CAD build for the part. Positions are in the model's coordinates, mm. Face numbers are marked on the shaded views. A direction names the side the tool comes from. Give positions to 0.01 mm unless a question says otherwise; leave off trailing zeros. Write each loop counter-clockwise with the first axis right and the second up, starting at its lowest first coordinate (ties: lowest second). Pieces come first, ordered by that corner, then holes. Notation, with made-up numbers: (85, -7.5) - (105, -7.5) arc R34 cw to (105, 23.5) - close; hole circle Ø3 at (-11, 85). An arc over 180 degrees is marked (long way). Put each result on its own line as item: value. Start each with the question number.
1. Tool access for the marked faces 4, 5 and 6: list every direction of +Z, -Z, +X, -X, +Y, -Y with a clear straight run to the whole face (end or side of a thin tool).
2. Mould opens along Y. For the marked faces 1, 2 and 3 say: +Y half, -Y half, draft (parallel to the pull), parting line (faces both ways), or undercut.
3. Drop flat-ended pins along their axis: pin 1 (2 mm diameter, centred on x = 5, z = 1.5, fed in from +Y); pin 2 (2 mm diameter, centred on x = -2.5, y = 4.5, fed in from +Z); pin 3 (8 mm diameter, centred on x = 4.5, y = 28.5, fed in from +Z); pin 4 (7 mm diameter, centred on y = 53.5, z = 0, fed in from +X). Give the stop position or say it passes through.
4. Cut at B-B on z = -4.25. List the corners of the cut face in (x, y), and give its area (3 significant figures).
5. Cut at D-D on y = 13.5. List the corners of the cut face in (x, z), and give its area (3 significant figures).
6. Cut at C-C on x = 3.25. List the corners of the cut face in (y, z), and give its area (3 significant figures).
7. Wall check: line 1 (Y direction, x = 5.2, z = 0); line 2 (Z direction, x = 3.65, y = 53.5); line 3 (Y direction, x = 6.25, z = 4.25). Give the ranges that are in metal, low to high.
8. Cut at A-A on x = -4.5. List the corners of the cut face in (y, z).
from build123d import *

# Parameters (mm, degrees)
SKETCH1_R           = 7.5
BOSS_EXTRUDE1_DEPTH = 46
SKETCH2_W           = 15
SKETCH2_H           = 15
BOSS_EXTRUDE2_DEPTH = 10
SKETCH3_R           = 2.5
CUT_EXTRUDE1_DEPTH  = 7.5
BOSS_EXTRUDE3_DEPTH = 15
CUT_EXTRUDE4_DEPTH  = 64.263338514
SKETCH6_R           = 6
CUT_EXTRUDE5_DEPTH  = 64.263338514
CUT_EXTRUDE7_START  = -5
SKETCH7_R           = 7.5
CUT_EXTRUDE7_DEPTH  = 5
CUT_EXTRUDE8_START  = -5
CUT_EXTRUDE8_DEPTH  = 5


with BuildPart() as part:
    # Sketch1 → Boss-Extrude1 (new body)
    with BuildSketch(Plane(origin=(0, 0, 0), x_dir=(1, 0, 0), z_dir=(0, 1, 0))):
        with Locations(Location((0, 0, 0), (0, 0, 270))):
            Circle(SKETCH1_R)
    extrude(amount=BOSS_EXTRUDE1_DEPTH)

    # Sketch2 → Boss-Extrude2 (add)
    with BuildSketch(Plane.XZ):
        Rectangle(SKETCH2_W, SKETCH2_H)
    extrude(amount=BOSS_EXTRUDE2_DEPTH)

    # Sketch3 → Cut-Extrude1 (cut)
    with BuildSketch(Plane.ZY.offset(7.5)):
        with Locations((0, -5)):
            Circle(SKETCH3_R)
    extrude(amount=-CUT_EXTRUDE1_DEPTH, mode=Mode.SUBTRACT)

    # Sketch4 → Boss-Extrude3 (add)
    with BuildSketch(Plane(origin=(0, 46, 0), x_dir=(1, 0, 0), z_dir=(0, 1, 0))):
        Polygon((0, 7.5), (7.5, 7.5), (7.5, -7.5), (-7.5, -7.5), (-7.5, 7.5), align=None)
    extrude(amount=BOSS_EXTRUDE3_DEPTH)

    # Sketch5 → Cut-Extrude4 (cut, through all)
    with BuildSketch(Plane.ZY.offset(7.5)):
        with BuildLine():
            ThreePointArc((-7.5, 53.5), (-5.303300859, 58.803300859), (0, 61))
            Line((0, 61), (-7.5, 61))
            Line((-7.5, 61), (-7.5, 53.5))
        make_face()
        with BuildLine():
            Line((7.5, 61), (0, 61))
            ThreePointArc((0, 61), (5.303300859, 58.803300859), (7.5, 53.5))
            Line((7.5, 53.5), (7.5, 61))
        make_face()
    extrude(amount=-CUT_EXTRUDE4_DEPTH, mode=Mode.SUBTRACT)

    # Sketch6 → Cut-Extrude5 (cut, through all)
    with BuildSketch(Plane.ZY.offset(7.5)):
        with Locations((0, 53.5)):
            Circle(SKETCH6_R)
    extrude(amount=-CUT_EXTRUDE5_DEPTH, mode=Mode.SUBTRACT)

    # Sketch7 → Cut-Extrude7 (cut)
    with BuildSketch(Plane.ZY.offset(7.5).offset(CUT_EXTRUDE7_START)):
        with Locations((0, 53.5)):
            Circle(SKETCH7_R)
    extrude(amount=-CUT_EXTRUDE7_DEPTH, mode=Mode.SUBTRACT)

    # Sketch8 → Cut-Extrude8 (cut)
    with BuildSketch(Plane.ZY.offset(7.5).offset(CUT_EXTRUDE8_START)):
        with BuildLine():
            Line((-6, 53.5), (-7.5, 53.5))
            Line((-7.5, 53.5), (-7.5, 46))
            Line((-7.5, 46), (0, 46))
            Line((0, 46), (7.5, 46))
            Line((7.5, 46), (7.5, 53.5))
            Line((7.5, 53.5), (6, 53.5))
            ThreePointArc((6, 53.5), (0, 47.5), (-6, 53.5))
        make_face()
    extrude(amount=-CUT_EXTRUDE8_DEPTH, mode=Mode.SUBTRACT)


solid = part.part
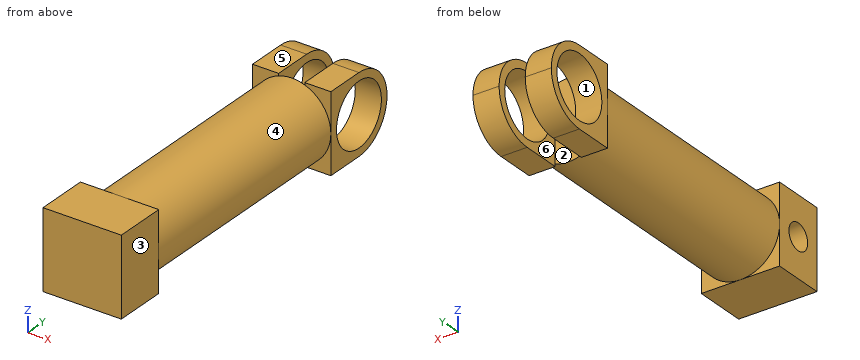
Report:
1. face 4: none
1. face 5: +Z, +X, -X, +Y, -Y
1. face 6: +Z, -Z, +Y
2. face 1: undercut
2. face 2: +Y half
2. face 3: draft
3. pin 1: stops at y = 60.98
3. pin 2: stops at z = 7.35
3. pin 3: stops at z = 7.48
3. pin 4: passes through
4. outline: (-7.5, -10) - (7.5, -10) - (7.5, 0) - (6.18, 0) - (6.18, 46) - (7.5, 46) - (7.5, 49.26) - (2.5, 49.26) - (2.5, 46) - (-2.5, 46) - (-2.5, 49.26) - (-7.5, 49.26) - (-7.5, 46) - (-6.18, 46) - (-6.18, 0) - (-7.5, 0) - close; (-7.5, 57.74) - (-2.5, 57.74) - (-2.5, 59.68) - (-7.5, 59.68) - close; (2.5, 57.74) - (7.5, 57.74) - (7.5, 59.68) - (2.5, 59.68) - close
4. area: 771 mm²
5. outline: circle Ø15 at (0, 0)
5. area: 177 mm²
6. outline: (-10, -7.5) - (0, -7.5) - (0, -6.76) - (46, -6.76) - (46, -7.5) - (53.5, -7.5) arc R7.5 ccw to (53.5, 7.5) - (46, 7.5) - (46, 6.76) - (0, 6.76) - (0, 7.5) - (-10, 7.5) - close; hole circle Ø12 at (53.5, 0)
6. area: 860 mm²
7. line 1: y = -10 to 47.5, 59.5 to 61
7. line 2: z = -7.5 to -6, 6 to 7.5
7. line 3: y = -10 to 0, 46 to 49.26, 57.74 to 59.68
8. outline: (-10, -7.5) - (0, -7.5) - (0, -6) - (46, -6) - (46, -7.5) - (53.5, -7.5) arc R7.5 ccw to (53.5, 7.5) - (46, 7.5) - (46, 6) - (0, 6) - (0, 7.5) - (-10, 7.5) - close; hole circle Ø5 at (-5, 0); hole circle Ø12 at (53.5, 0)
